Can you work these out from the model? Positions are in its coordinate system, mm. Give positions to 0.01 mm unless a question says otherwise; leave off trailing zeros. Loops run counter-clockwise (first coordinate to the right, second up) from the corner with the lowest first, then second, coordinate; pieces in that order, holes last. Notation, with made-up numbers: (-19.75, 3.5) -> (-7.75, 3.5) arc R25 cw to (-7.75, 26.5) -> close; hole circle Ø6 at (23, 73). An arc over 180 degrees is marked (long way). Return JSON: item names as keys, results as strings. Group by question number.
Q1. Suppose I cut it at A-A, the plane x = -7.5. Please give me the cut outline in (y, z), and give its area (3 significant figures).
Q2. I need wall thicknesses on line 1 along Y through (x, z) = (58.5, 1.65); line 2 along Y through (x, z) = (73, 3); line 3 along X through (y, z) = (91.5, 1.6). Which ranges of each line are inside material? Lowest first, please. Write a range as [from, to].
Q3. Will these pins go through, and if not, where does the flat tip stop? pin 1 (1.5 mm diameter, centred on x = 32.5, z = 1.5, fed in from -Y); pin 2 (1.2 mm diameter, centred on y = -124.5, z = 2.5, fed in from +X); pin 3 (2 mm diameter, centred on x = 42.5, z = 1.5, fed in from +Y); pin 4 (2 mm diameter, centred on x = -25, y = 39.5, fed in from -Z).
Q4. Suppose I cut it at B-B, the plane y = 140.5. Count the separate pieces of the cut face and the enclosed holes in it, and give its area (3 significant figures).
Q5. Suppose I cut it at D-D, the plane y = -106. Please give me the cut outline in (x, z), and give its area (3 significant figures).
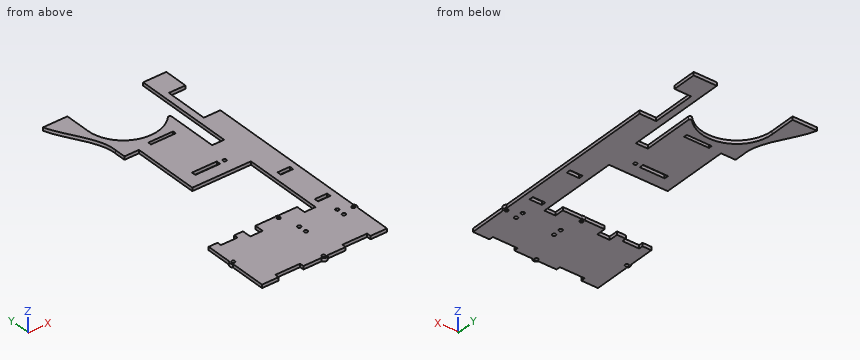
```python
from build123d import *

# Parameters (mm, degrees)
SKETCH1_W           = 151
SKETCH1_H           = 254
BOSS_EXTRUDE1_DEPTH = 4
SKETCH2_W           = 49.486524855
SKETCH2_H           = 99.222786378
CUT_EXTRUDE1_DEPTH  = 5
SKETCH4_W           = 120.35
SKETCH4_H           = 88.04721362
CUT_EXTRUDE3_DEPTH  = 5
SKETCH6_R           = 2
CUT_EXTRUDE5_DEPTH  = 10
SKETCH12_W          = 15
SKETCH12_H          = 10
SKETCH12_W_2        = 13.35
CUT_EXTRUDE8_DEPTH  = 10
SKETCH13_R          = 2
CUT_EXTRUDE9_DEPTH  = 5
SKETCH14_R          = 4
SKETCH14_R_2        = 2
BOSS_EXTRUDE2_DEPTH = 4
SKETCH15_R          = 2.1
CUT_EXTRUDE10_DEPTH = 10
SKETCH18_R          = 2
CUT_EXTRUDE12_DEPTH = 5
SKETCH19_R          = 4
SKETCH19_R_2        = 2
BOSS_EXTRUDE3_DEPTH = 4
SKETCH25_W          = 59.513475145
SKETCH25_H          = 4
CUT_EXTRUDE16_DEPTH = 10
SKETCH26_W          = 151
SKETCH26_H          = 86
BOSS_EXTRUDE4_DEPTH = 4
SKETCH27_W          = 42
SKETCH27_H          = 62
BOSS_EXTRUDE5_DEPTH = 4
CUT_EXTRUDE17_DEPTH = 5
SKETCH29_W          = 20
SKETCH29_H          = 53
CUT_EXTRUDE18_DEPTH = 10
SKETCH30_W          = 14.513475145
SKETCH30_H          = 123
CUT_EXTRUDE19_DEPTH = 10
CUT_EXTRUDE20_DEPTH = 10
FILLET1_R           = 2
SKETCH33_W          = 30
SKETCH33_H          = 4
CUT_EXTRUDE22_DEPTH = 10
SKETCH34_W          = 30
SKETCH34_H          = 5
SKETCH34_W_2        = 15
CUT_EXTRUDE23_DEPTH = 10
SKETCH35_W          = 50.5
SKETCH35_H          = 0.999999998
SKETCH35_W_2        = 41.5
BOSS_EXTRUDE6_DEPTH = 4
SKETCH36_W          = 20.104648663
SKETCH36_H          = 5
CUT_EXTRUDE24_DEPTH = 5
SKETCH37_R          = 2
CUT_EXTRUDE25_DEPTH = 5
SKETCH38_R          = 4
SKETCH38_R_2        = 2
BOSS_EXTRUDE7_DEPTH = 4
SKETCH39_R          = 2
CUT_EXTRUDE26_DEPTH = 10


with BuildPart() as part:
    # Sketch1 → Boss-Extrude1 (new body)
    with BuildSketch(Plane.XY):
        with Locations((0, 0.5)):
            Rectangle(SKETCH1_W, SKETCH1_H)
    extrude(amount=BOSS_EXTRUDE1_DEPTH)

    # Sketch2 → Cut-Extrude1 (cut)
    with BuildSketch(Plane.XY.offset(4)):
        with Locations((-50.756737573, 77.888606811)):
            Rectangle(SKETCH2_W, SKETCH2_H)
    extrude(amount=-CUT_EXTRUDE1_DEPTH, mode=Mode.SUBTRACT)

    # Sketch4 → Cut-Extrude3 (cut)
    with BuildSketch(Plane.XY.offset(4)):
        with Locations((-15.325, -2.476393188)):
            Rectangle(SKETCH4_W, SKETCH4_H)
    extrude(amount=-CUT_EXTRUDE3_DEPTH, mode=Mode.SUBTRACT)

    # Sketch6 → Cut-Extrude5 (cut)
    with BuildSketch(Plane.XY.offset(4)):
        with Locations((0, -125)):
            Circle(SKETCH6_R)
    extrude(amount=-CUT_EXTRUDE5_DEPTH, mode=Mode.SUBTRACT)

    # Sketch12 → Cut-Extrude8 (cut)
    with BuildSketch(Plane.XY.offset(4)):
        with Locations((-26.5, -51.499999998)):
            Rectangle(SKETCH12_W, SKETCH12_H)
        with Locations((38.175, -51.499999998)):
            Rectangle(SKETCH12_W_2, SKETCH12_H)
    extrude(amount=-CUT_EXTRUDE8_DEPTH, mode=Mode.SUBTRACT)

    # Sketch13 → Cut-Extrude9 (cut)
    with BuildSketch(Plane.XY.offset(4)):
        with Locations((6.25, -49)):
            Circle(SKETCH13_R)
    extrude(amount=-CUT_EXTRUDE9_DEPTH, mode=Mode.SUBTRACT)

    # Sketch14 → Boss-Extrude2 (add)
    # profile 1 of 2: a face of its own
    with BuildSketch(Plane.XY.offset(4)):
        with Locations((6.25, -49)):
            Circle(SKETCH14_R)
        with Locations((6.25, -49)):
            Circle(SKETCH14_R_2, mode=Mode.SUBTRACT)
    # profile 2 of 2: a face of its own
    with BuildSketch(Plane.XY.offset(4)):
        with Locations((0, -125)):
            Circle(SKETCH14_R)
        with Locations((0, -125)):
            Circle(SKETCH14_R_2, mode=Mode.SUBTRACT)
    extrude(amount=-BOSS_EXTRUDE2_DEPTH)

    # Sketch15 → Cut-Extrude10 (cut)
    with BuildSketch(Plane(origin=(0, 0, 0), x_dir=(-1, 0, 0), z_dir=(0, 0, -1))):
        with Locations((-58.5, -72.5)):
            Circle(SKETCH15_R)
        with Locations((-58.5, -82.5)):
            Circle(SKETCH15_R)
        with Locations((-12.5, -72.5)):
            Circle(SKETCH15_R)
        with Locations((-12.5, -82.5)):
            Circle(SKETCH15_R)
    extrude(amount=-CUT_EXTRUDE10_DEPTH, mode=Mode.SUBTRACT)

    # Sketch18 → Cut-Extrude12 (cut)
    with BuildSketch(Plane.XY.offset(4)):
        with Locations((-73, -79.562158061)):
            Circle(SKETCH18_R)
    extrude(amount=-CUT_EXTRUDE12_DEPTH, mode=Mode.SUBTRACT)

    # Sketch19 → Boss-Extrude3 (add)
    with BuildSketch(Plane.XY.offset(4)):
        with Locations((-73, -79.562158061)):
            Circle(SKETCH19_R)
        with Locations((-73, -79.562158061)):
            Circle(SKETCH19_R_2, mode=Mode.SUBTRACT)
    extrude(amount=-BOSS_EXTRUDE3_DEPTH)

    # Sketch25 → Cut-Extrude16 (cut)
    with BuildSketch(Plane.XY.offset(4)):
        with Locations((3.743262427, 124.5)):
            Rectangle(SKETCH25_W, SKETCH25_H)
    extrude(amount=-CUT_EXTRUDE16_DEPTH, mode=Mode.SUBTRACT)

    # Sketch26 → Boss-Extrude4 (add)
    with BuildSketch(Plane.XY.offset(4)):
        with Locations((0, 165.5)):
            Rectangle(SKETCH26_W, SKETCH26_H)
    extrude(amount=-BOSS_EXTRUDE4_DEPTH)

    # Sketch27 → Boss-Extrude5 (add)
    with BuildSketch(Plane.XY.offset(4)):
        with Locations((54.5, 91.5)):
            Rectangle(SKETCH27_W, SKETCH27_H)
    extrude(amount=-BOSS_EXTRUDE5_DEPTH)

    # Sketch28 → Cut-Extrude17 (cut)
    with BuildSketch(Plane(origin=(0, 0, 0), x_dir=(-1, 0, 0), z_dir=(0, 0, -1))):
        with BuildLine():
            Line((43.55584756, 136.203397333), (43.55584756, 122.5))
            Line((43.55584756, 122.5), (75.5, 122.5))
            Line((75.5, 122.5), (75.5, 208.5))
            Line((75.5, 208.5), (73.5, 208.5))
            add(Edge.make_bspline(
                [(73.5, 208.5), (66.265840294, 185.251616354), (42.071208011, 161.186737721), (43.55584756, 136.203397333)],
                knots=[0, 0, 0, 0, 0.885856011, 0.885856011, 0.885856011, 0.885856011], degree=3))
        make_face()
    extrude(amount=-CUT_EXTRUDE17_DEPTH, mode=Mode.SUBTRACT)

    # Sketch29 → Cut-Extrude18 (cut)
    with BuildSketch(Plane(origin=(0, 0, 0), x_dir=(-1, 0, 0), z_dir=(0, 0, -1))):
        with Locations((-65.5, 153)):
            Rectangle(SKETCH29_W, SKETCH29_H)
    extrude(amount=-CUT_EXTRUDE18_DEPTH, mode=Mode.SUBTRACT)

    # Sketch30 → Cut-Extrude19 (cut)
    with BuildSketch(Plane.XY.offset(4)):
        with Locations((40.243262427, 147)):
            Rectangle(SKETCH30_W, SKETCH30_H)
    extrude(amount=-CUT_EXTRUDE19_DEPTH, mode=Mode.SUBTRACT)

    # Sketch31 → Cut-Extrude20 (cut)
    with BuildSketch(Plane.XY.offset(4)):
        with BuildLine():
            Line((-44, 177.3), (-44, 208.5))
            Line((-44, 208.5), (41, 208.5))
            Line((41, 208.5), (41, 177.3))
            ThreePointArc((41, 177.3), (-1.5, 134.8), (-44, 177.3))
        make_face()
    extrude(amount=-CUT_EXTRUDE20_DEPTH, mode=Mode.SUBTRACT)

    # Fillet1
    fillet1_edges = [part.edges().sort_by_distance(p)[0] for p in [
        (32.986524855, 152.461932373, 2),
    ]]
    fillet(fillet1_edges, radius=FILLET1_R)

    # Sketch33 → Cut-Extrude22 (cut)
    with BuildSketch(Plane.XY.offset(4)):
        with Locations((3.5, 124.5)):
            Rectangle(SKETCH33_W, SKETCH33_H)
    extrude(amount=-CUT_EXTRUDE22_DEPTH, mode=Mode.SUBTRACT)

    # Sketch34 → Cut-Extrude23 (cut)
    with BuildSketch(Plane.XY.offset(4)):
        with Locations((40.5, -124)):
            Rectangle(SKETCH34_W, SKETCH34_H)
        with Locations((-40.5, -124)):
            Rectangle(SKETCH34_W, SKETCH34_H)
        with Locations((60.175, -48)):
            Rectangle(SKETCH34_W_2, SKETCH34_H)
        with Locations((60.5, 9)):
            Rectangle(SKETCH34_W_2, SKETCH34_H)
        with Locations((4.5, 59)):
            Rectangle(SKETCH34_W, SKETCH34_H)
    extrude(amount=-CUT_EXTRUDE23_DEPTH, mode=Mode.SUBTRACT)

    # Sketch35 → Boss-Extrude6 (add)
    with BuildSketch(Plane.XY.offset(4)):
        with Locations((6.25, -45.999999999)):
            Rectangle(SKETCH35_W, SKETCH35_H)
        with Locations((-54.75, -45.999999999)):
            Rectangle(SKETCH35_W_2, SKETCH35_H)
    extrude(amount=-BOSS_EXTRUDE6_DEPTH)

    # Sketch36 → Cut-Extrude24 (cut)
    with BuildSketch(Plane.XY.offset(4)):
        with Locations((-54.697675668, -48)):
            Rectangle(SKETCH36_W, SKETCH36_H)
    extrude(amount=-CUT_EXTRUDE24_DEPTH, mode=Mode.SUBTRACT)

    # Sketch37 → Cut-Extrude25 (cut)
    with BuildSketch(Plane.XY.offset(4)):
        with Locations((73, -78.562158061)):
            Circle(SKETCH37_R)
    extrude(amount=-CUT_EXTRUDE25_DEPTH, mode=Mode.SUBTRACT)

    # Sketch38 → Boss-Extrude7 (add)
    with BuildSketch(Plane.XY.offset(4)):
        with Locations((73, -78.562158061)):
            Circle(SKETCH38_R)
        with Locations((73, -78.562158061)):
            Circle(SKETCH38_R_2, mode=Mode.SUBTRACT)
    extrude(amount=-BOSS_EXTRUDE7_DEPTH)

    # Sketch39 → Cut-Extrude26 (cut)
    with BuildSketch(Plane.XY.offset(4)):
        with Locations((26.57851787, 58.5)):
            Circle(SKETCH39_R)
    extrude(amount=-CUT_EXTRUDE26_DEPTH, mode=Mode.SUBTRACT)


solid = part.part
```
Ans:
{
 "1": {"outline": "(-126.5, 0) -> (-45.5, 0) -> (-45.5, 4) -> (-126.5, 4) -> close; (41.55, 0) -> (56.5, 0) -> (56.5, 4) -> (41.55, 4) -> close; (61.5, 0) -> (122.5, 0) -> (122.5, 4) -> (61.5, 4) -> close; (126.5, 0) -> (135.23, 0) -> (135.23, 4) -> (126.5, 4) -> close", "area": "663 mm^2"},
 "2": {"line 1": "y = [-126.5, -84.6], [-80.4, -74.6], [-70.4, -50.5], [-45.5, 6.5], [11.5, 126.5], [179.5, 208.5]", "line 2": "y = [-126.5, -80.56], [-76.56, 126.5], [179.5, 208.5]", "line 3": "x = [-26.01, 32.99], [47.5, 75.5]"},
 "3": {"pin 1": "stops at y = -121.5", "pin 2": "stops at x = 75.5", "pin 3": "stops at y = 85.5", "pin 4": "passes through"},
 "4": {"separate pieces": "3", "enclosed holes": "0", "area": "168 mm^2"},
 "5": {"outline": "(-75.5, 0) -> (75.5, 0) -> (75.5, 4) -> (-75.5, 4) -> close", "area": "604 mm^2"}
}
